Job drawing, mm, ordinate dimensions from the low corner. One solid piece. Give positions to 0.01 mm unless a question says otherwise; leave off trailing zeros. Loops run counter-clockwise (first coordinate to the right, second up) from the corner with the lowest first, then second, coordinate; pieces in that order, holes last. Notation, with made-up numbers: (-4, 63) -> (6, 63) arc R27 cw to (6, 82) -> close; hole circle Ø8 at (77.5, 16.25). An arc over 180 degrees is marked (long way). Answer as a JSON object with one key per item and string values. Group by question number.
Q1. Band-saw the part on D-D, the plane x = 4. Write the cut outline in (y, z) (1 decimal), plus the area to 3 significant figures.
Q2. Band-saw the part on C-C, the plane z = 0.65. Count the separate pieces of the cut face and the enclosed holes in it, plus the area to 3 significant figures.
Q3. Band-saw the part on B-B, the plane x = 31.3. Write the cut outline in (y, z) (1 decimal), plus the area to 3 significant figures.
Q4. Wall check: probe 1 along Y at (x, z) = (6.3, 0.7); probe 2 along Y at (x, z) = (4, 0.6); probe 3 along X at (y, z) = (29.5, 0.45). Give the ranges that are in metal, low to high. Write a range as from..to.
Q5. Band-saw the part on A-A, the plane y = 12.7. Write the cut outline in (x, z) (1 decimal), plus the area to 3 significant figures.
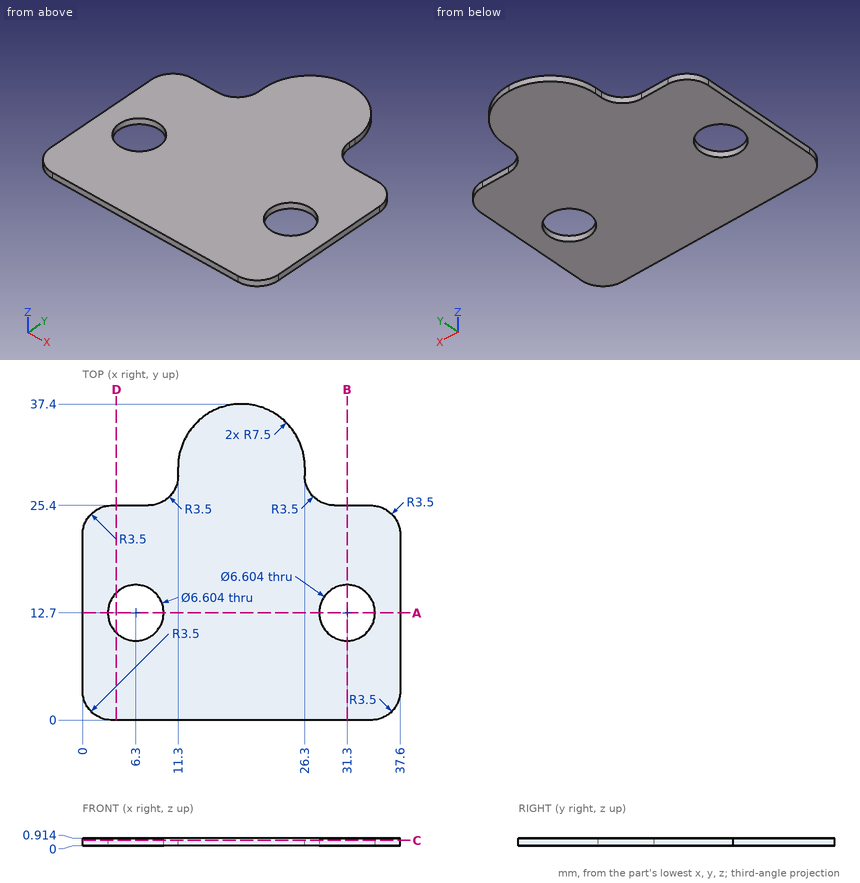
Worked answers:
{
 "1": {"outline": "(0, 0) -> (10.3, 0) -> (10.3, 0.9) -> (0, 0.9) -> close; (15.1, 0) -> (25.4, 0) -> (25.4, 0.9) -> (15.1, 0.9) -> close", "area": "18.9 mm2"},
 "2": {"separate pieces": "1", "enclosed holes": "2", "area": "1,040 mm2"},
 "3": {"outline": "(0, 0) -> (9.4, 0) -> (9.4, 0.9) -> (0, 0.9) -> close; (16, 0) -> (25.4, 0) -> (25.4, 0.9) -> (16, 0.9) -> close", "area": "17.2 mm2"},
 "4": {"probe 1": "0..9.4, 16..25.4", "probe 2": "0..10.33, 15.07..25.4", "probe 3": "11.3..26.3"},
 "5": {"outline": "(0, 0) -> (3, 0) -> (3, 0.9) -> (0, 0.9) -> close; (9.6, 0) -> (28, 0) -> (28, 0.9) -> (9.6, 0.9) -> close; (34.6, 0) -> (37.6, 0) -> (37.6, 0.9) -> (34.6, 0.9) -> close", "area": "22.3 mm2"}
}
